Geometry: see drawing. Coordinates: mm, zero at the bounding-box minimum. A direction names the side the tool comes from. Round coordinates to 2 decimals unless told otherwise and drop trailing zeros. Write each loop counter-clockwise with the first axis right and the second up, starting at its lowest first coordinate (ties: lowest second). Pieces come first, ordered by that corner, then holes.
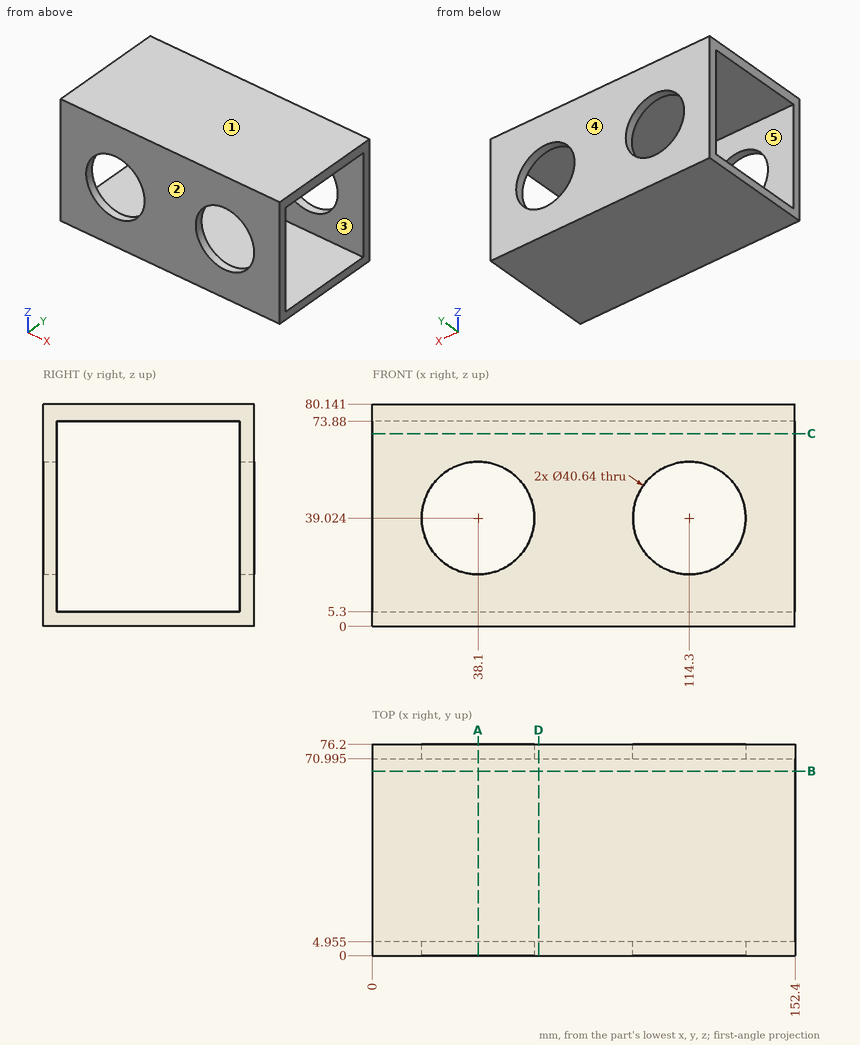
1) Contact query for flat-ended pins moving along their axis: P1, Ø2, axis at x = 79, y = 28.5, coming from the -Z side; P2, Ø24.5, axis at x = 38.1, z = 39.02, coming from the +Y side. Output: stop coordinate, or through.
Taken from the geometry:
P1: stops at z = 0
P2: passes through
2) Pull-direction query (Y, two-part tool) for the marked faces 1, 2 and 3; classes: released by +Y, released by -Y, zero draft, split by the parting line, or undercut.
Taken from the geometry:
face 1: zero draft
face 2: released by -Y
face 3: undercut
3) Section query C-C on z = 69.5. Return the cut outline in (x, y) (1 decimal), then the cut area to 3 significant figures.
Taken from the geometry:
outline: (0, 0) - (152.4, 0) - (152.4, 5) - (0, 5) - close; (0, 71) - (152.4, 71) - (152.4, 76.2) - (0, 76.2) - close
area: 1,550 mm2
4) Section query B-B on y = 66.5. Return the cut outline in (x, z), then the cut area to 3 significant figures.
Taken from the geometry:
outline: (0, 0) - (152.4, 0) - (152.4, 5.3) - (0, 5.3) - close; (0, 73.88) - (152.4, 73.88) - (152.4, 80.14) - (0, 80.14) - close
area: 1,760 mm2
5) Material intervals for line 1 (Z direction, x = 38, y = 3) (1 decimal); line 2 (Y direction, x = 42.5, z = 6.5) (1 decimal); line 3 (Z direction, x = 145.5, y = 43.5), sorted ascending.
Taken from the geometry:
line 1: z = 0 to 18.7, 59.3 to 80.1
line 2: y = 0 to 5, 71 to 76.2
line 3: z = 0 to 5.3, 73.88 to 80.14
6) Reachability of the marked faces 4 and 5 from +Z, -Z, +X, -X, +Y, -Y: full face, straight path, thin tool, end or side. Return the list, or none.
Taken from the geometry:
face 4: +Z, -Z, +X, -X, +Y
face 5: +X, -X
7) Section query A-A on x = 38.1. Return the cut outline in (y, z) (1 decimal).
Taken from the geometry:
outline: (0, 0) - (76.2, 0) - (76.2, 18.7) - (71, 18.7) - (71, 5.3) - (5, 5.3) - (5, 18.7) - (0, 18.7) - close; (0, 59.3) - (5, 59.3) - (5, 73.9) - (71, 73.9) - (71, 59.3) - (76.2, 59.3) - (76.2, 80.1) - (0, 80.1) - close
8) Section query D-D on x = 60. Return the cut outline in (y, z) (1 decimal), then the cut area to 3 significant figures.
Taken from the geometry:
outline: (0, 0) - (76.2, 0) - (76.2, 80.1) - (0, 80.1) - close; hole (5, 5.3) - (71, 5.3) - (71, 73.9) - (5, 73.9) - close
area: 1,580 mm2
